```python
from build123d import *

# Parameters (mm, degrees)
F2_DEPTH = 720
F1_W     = 600
F1_H     = 550
F3_DEPTH = 18
F5_DEPTH = 140


with BuildPart() as f2:
    # F0 (on Top) → F2 (new body)
    with BuildSketch(Plane.XY):
        Polygon((81.165642, 504.102758), (-518.834358, 504.102758), (-518.834358, -45.897242), (-500.834358, -45.897242), (-500.834358, 501.102758), (63.165642, 501.102758), (63.165642, -45.897242), (81.165642, -45.897242), align=None)
    extrude(amount=F2_DEPTH)

    # F1 (on Top) → F3 (join)
    with BuildSketch(Plane.XY):
        with Locations((-218.834358, 229.102758)):
            Rectangle(F1_W, F1_H)
    extrude(amount=F3_DEPTH)

    # F4 (on Top) → F5 (join)
    with BuildSketch(Plane.XY):
        Polygon((81.165642, 504.102758), (-518.834358, 504.102758), (-518.834358, -45.897242), (-500.834358, -45.897242), (-500.834358, 4.102758), (63.165642, 4.102758), (63.165642, -45.897242), (81.165642, -45.897242), align=None)
    extrude(amount=-F5_DEPTH)


solid = f2.part
```
Model file for the job. Use its own axes, mm. A direction names the side the tool comes from. Coordinates: 2 decimals unless noted, no trailing zeros. Order: outer loops, then holes, each group sorted by start corner. A loop starts at its lowest first (then second) coordinate and runs counter-clockwise, first axis right, second up. Notation, with made-up numbers: M 51.25,4.5 L 92.25,4.5 A34 ccw 92.25,36.5 Z; hole C 3,23 d8. An arc over 180 degrees is marked long. Answer as CSV lines item,"result".
(1) Band-saw the part on A-A, the plane y = 86. List the corners of the cut face in (x, z), then the cut area to 3 significant figures.
Geometry says:
outline,"M -518.83,-140 L 81.17,-140 L 81.17,720 L 63.17,720 L 63.17,18 L -500.83,18 L -500.83,720 L -518.83,720 Z"
area,"120,000 mm2"
(2) Pull direction X, two halves, no side cores. Call faces 4 (the flat face through (-500.834, 224, 364)), 5 (the flat face through (-215, 504.103, 296)), 6 (the flat face through (-518.834, 233, 296)): +X half, -X half, draft (parallel to the pull), parting line (faces both ways), or undercut.
Geometry says:
face 4,"undercut"
face 5,"draft"
face 6,"-X half"
(3) Wall check: line 1 along X through (y, z) = (210, 431); line 2 along Z through (x, y) = (-11, 61); line 3 along Y through (x, z) = (51, 497). Give the ranges that are in metal, low to high.
Geometry says:
line 1,"x = -518.83 to -500.83, 63.17 to 81.17"
line 2,"z = -140 to 18"
line 3,"y = 501.1 to 504.1"
(4) 3-axis set-ups, long thin cutter, end or side, ignore diameter. For faces 1 (the flat face through (-223, 501.103, 364)), 2 (the flat face through (-500.834, -21, -69)), 3 (the flat face through (-220, -45.897, 5)): which of +Z, -Z, +X, -X, +Y, -Y reach the whole face in a straight line?
Geometry says:
face 1,"+Z, -Y"
face 2,"-Z, -Y"
face 3,"+Z, -Z, +X, -X, -Y"
(5) Band-saw the part on B-B, the plane z = 152.5. List the corners of the cut face in (x, y), then the cut area to 3 significant figures.
Geometry says:
outline,"M -518.83,-45.9 L -500.83,-45.9 L -500.83,501.1 L 63.17,501.1 L 63.17,-45.9 L 81.17,-45.9 L 81.17,504.1 L -518.83,504.1 Z"
area,"21,500 mm2"
